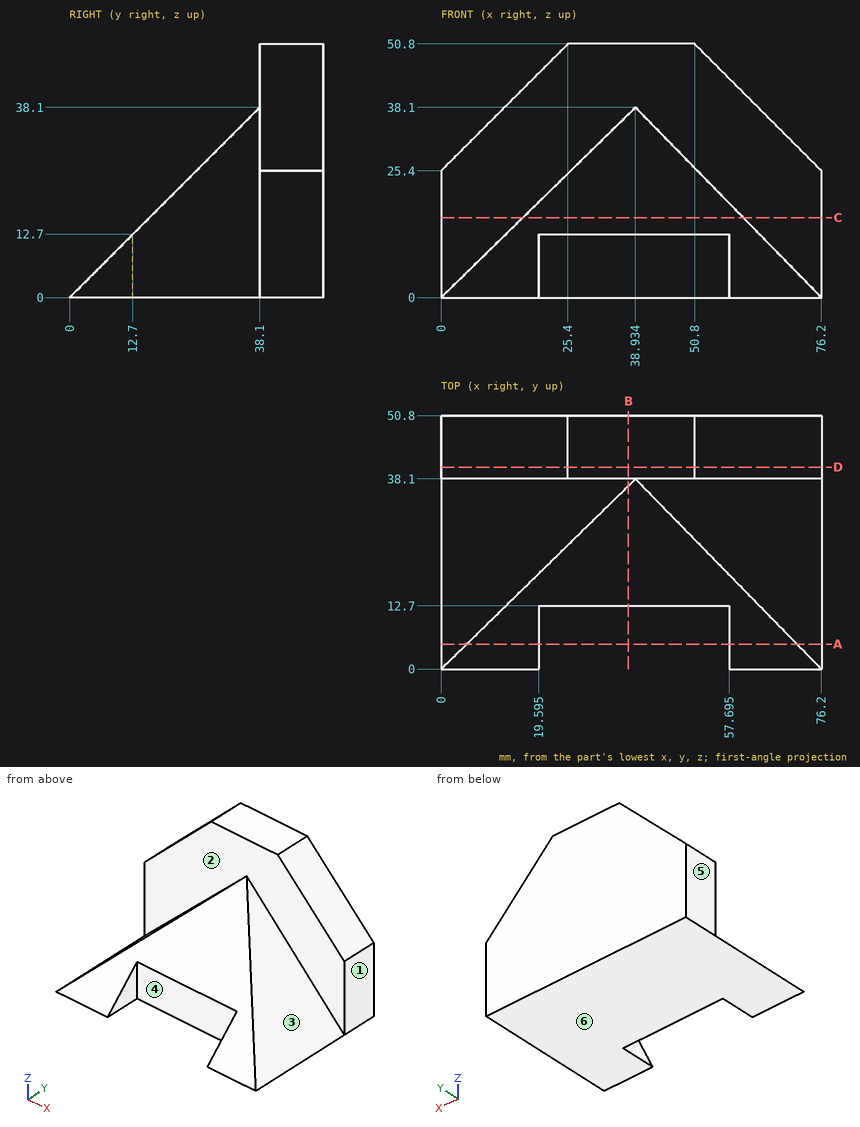
Input: dimensioned drawing with shaded views. Units: mm. Origin: part minimum x, y, z. A direction names the side the tool comes from. Give positions to 0.01 mm unless a question says otherwise; leave off trailing zeros. Loops run counter-clockwise (first coordinate to the right, second up) from the corner with the lowest first, then second, coordinate; pieces in that order, holes last. Notation, with made-up numbers: (38.5, 26) - (44.5, 26) arc R15 cw to (44.5, 34) - close; hole circle Ø10 at (-8, 83.5). An arc over 180 degrees is marked (long way). Answer as CSV lines item,"result". Start each with the question number.
(1) Section query C-C (z = 16). Output: boundary loops of the cut face in (x, y), and give its area (3 significant figures).
(2) Pin query (flat end, axial travel): P1, Ø6.5, axis at x = 39.5, z = 4.5, coming from the -Y side; P2, Ø10, axis at x = 16, z = 37, coming from the -Y side; P3, Ø1, axis at x = 34, y = 34.5, coming from the +Z side; P4, Ø2, axis at x = 57, y = 41, coming from the -Z side. Return the tip coordinate at first contact, or that it passes through.
(3) Mould query, pull axis X, two halves, no side actions, for the marked faces 3, 4, 5 and 6. Classes: +X half, -X half, draft (parallel to the pull), parting line (faces both ways), or undercut.
(4) Section query D-D (y = 40.5). Output: boundary loops of the cut face in (x, z).
(5) Section query A-A (y = 5). Output: boundary loops of the cut face in (x, z) (1 decimal).
(6) Section query B-B (x = 37.5). Output: boundary loops of the cut face in (y, z).
(7) Reachability of the marked faces 1 and 2 from +Z, -Z, +X, -X, +Y, -Y: full face, straight path, thin tool, end or side. Return the list, or none.
(8) Ray query, line 1 along Y through (x, z) = (39.5, 3.5); line 2 along Y through (x, z) = (62, 28); line 3 along X through (y, z) = (39, 43). Return the intervals inside material, ascending. Write a range as [from, to].
Worked answers:
1,outline,"(0, 38.1) - (16.35, 38.1) - (16.35, 16) - (60.55, 16) - (60.55, 38.1) - (76.2, 38.1) - (76.2, 50.8) - (0, 50.8) - close"
1,area,"1,940 mm^2"
2,P1,"stops at y = 12.7"
2,P2,"stops at y = 38.1"
2,P3,"stops at z = 33.76"
2,P4,"stops at z = 0"
3,face 3,"+X half"
3,face 4,"undercut"
3,face 5,"-X half"
3,face 6,"draft"
4,outline,"(0, 0) - (76.2, 0) - (76.2, 25.4) - (50.8, 50.8) - (25.4, 50.8) - (0, 25.4) - close"
5,outline,"(0, 0) - (19.6, 0) - (19.6, 5) - (5.1, 5) - close; (57.7, 0) - (76.2, 0) - (71.3, 5) - (57.7, 5) - close"
6,outline,"(12.7, 0) - (50.8, 0) - (50.8, 50.8) - (38.1, 50.8) - (38.1, 36.7) - (36.7, 36.7) - (12.7, 12.7) - close"
7,face 1,"+Z, -Z, +X, +Y, -Y"
7,face 2,"+Z, -Y"
8,line 1,"y = [12.7, 50.8]"
8,line 2,"y = [38.1, 50.8]"
8,line 3,"x = [17.6, 58.6]"
